The drawing under review shows one solid part. Ordinate dimensions are in mm from its lowest x, y, z. A direction names the side the tool comes from. Round coordinates to 2 decimals unless told otherwise and drop trailing zeros. Order: outer loops, then holes, each group sorted by start corner. A loop starts at its lowest first (then second) coordinate and runs counter-clockwise, first axis right, second up. Notation, with made-up numbers: (76, 42) -> (131, 42) arc R18 ccw to (131, 77) -> close; hole circle Ø2 at (77, 69). An arc over 180 degrees is marked (long way). Put each result on its own line as item: value. Start each with the question number.
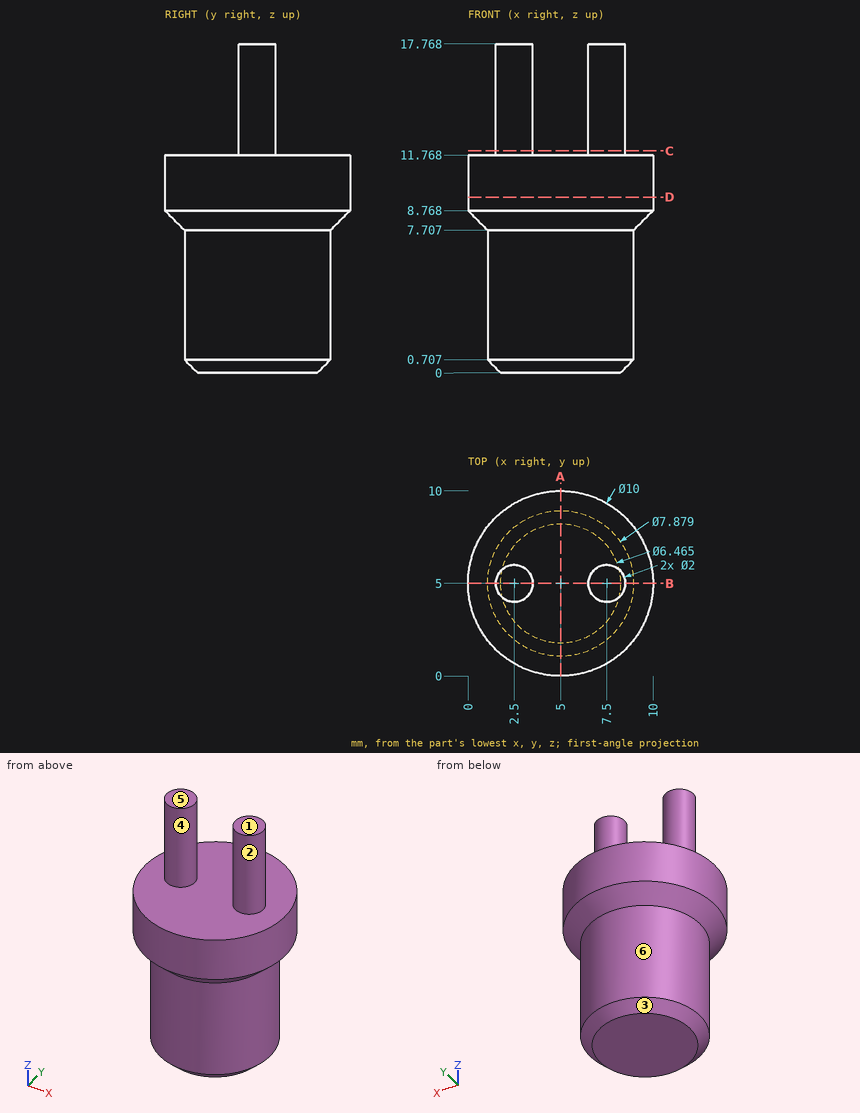
Item 1: Consider section A-A, the plane x = 5. Write out the cut boundary in (y, z).
Item 2: Consider section D-D, the plane z = 9.5. Write out the cut boundary in (x, y).
Item 3: Mouldability with a two-part tool opening along X and no side actions: class the marked faces 1, 2, 3 and 4 as +X half, -X half, draft (parallel to the pull), parting line (faces both ways), or undercut.
Item 4: Consider section B-B, the plane y = 5. Write out the cut boundary in (x, z).
Item 5: For L1, parallel to Z at x = 4.75, y = 5.75; L2, parallel to X at y = 5.5, z = 3.5, list the stretches that pass through material, from the lowest coordinate up.
Item 6: Tool access review of the marked faces 5 and 6: name each direction out of +Z, -Z, +X, -X, +Y, -Y from which nothing blocks a thin tool from reaching the whole face with its end or side.
Item 7: Consider section C-C, the plane z = 12. Write out the cut boundary in (x, y).
Item 8: Insertion check: pin 1 Ø1 at (x, y) = (4, 1.5) entering from +Z; pin 2 Ø1 at (x, z) = (3.5, 14.5) entering from -Y (1 decimal); pin 3 Ø3 at (x, z) = (5.5, 6.5) entering from -Y. Each pin has a flat end and moves straight along its axis. Give the tip position at first contact, or say it passes through.
Evaluation:
1. outline: (0, 8.77) -> (1.06, 7.71) -> (1.06, 0.71) -> (1.77, 0) -> (8.23, 0) -> (8.94, 0.71) -> (8.94, 7.71) -> (10, 8.77) -> (10, 11.77) -> (0, 11.77) -> close
2. outline: circle Ø10 at (5, 5)
3. face 1: draft
3. face 2: undercut
3. face 3: parting line
3. face 4: undercut
4. outline: (0, 8.77) -> (1.06, 7.71) -> (1.06, 0.71) -> (1.77, 0) -> (8.23, 0) -> (8.94, 0.71) -> (8.94, 7.71) -> (10, 8.77) -> (10, 11.77) -> (8.5, 11.77) -> (8.5, 17.77) -> (6.5, 17.77) -> (6.5, 11.77) -> (3.5, 11.77) -> (3.5, 17.77) -> (1.5, 17.77) -> (1.5, 11.77) -> (0, 11.77) -> close
5. L1: z = 0 to 11.77
5. L2: x = 1.09 to 8.91
6. face 5: +Z, +X, -X, +Y, -Y
6. face 6: -Z
7. outline: circle Ø2 at (2.5, 5); circle Ø2 at (7.5, 5)
8. pin 1: stops at z = 11.77
8. pin 2: stops at y = 4.1
8. pin 3: stops at y = 0.79
